from build123d import *

# Parameters (mm, degrees)
SKETCH_1_R               = 250
EXTRUDE_1_DEPTH          = 50
CHAMFER_1_SIZE           = 1
CUT_EXTRUDE_1_DEPTH      = 22
CUT_EXTRUDE_2_DEPTH      = 16
CUT_EXTRUDE_3_DEPTH      = 22
CUT_EXTRUDE_4_DEPTH      = 16
PATTERN_CIRCULAR_1_COUNT = 4
SKETCH_6_R               = 60
CUT_EXTRUDE_5_DEPTH      = 20
SKETCH_22_R              = 40
CUT_EXTRUDE_13_DEPTH     = 355.823899984


with BuildPart() as part:
    # Sketch 1 → Extrude 1 (new body)
    with BuildSketch(Plane(origin=(0, 0, 0), x_dir=(1, 0, 0), z_dir=(0, 1, 0))):
        with Locations(Location((0, 0, 0), (0, 0, 270))):
            Circle(SKETCH_1_R)
    extrude(amount=EXTRUDE_1_DEPTH)

    # Chamfer 1
    chamfer_1_edges = [part.edges().sort_by_distance(p)[0] for p in [
        (0, 0, -250),
        (0, 50, -250),
    ]]
    chamfer(chamfer_1_edges, length=CHAMFER_1_SIZE)

    # Sketch 2 → Cut-Extrude 1 (cut)
    with BuildSketch(Plane(origin=(0, 50, 0), x_dir=(1, 0, 0), z_dir=(0, 1, 0))):
        with BuildLine():
            Line((125, 11), (250, 11))
            Line((250, 11), (250, -11))
            Line((250, -11), (125, -11))
            ThreePointArc((125, -11), (114, 0), (125, 11))
        make_face()
    cut_extrude_1 = extrude(amount=-CUT_EXTRUDE_1_DEPTH, mode=Mode.SUBTRACT)

    # Sketch 3 → Cut-Extrude 2 (cut)
    with BuildSketch(Plane(origin=(0, 28, 0), x_dir=(1, 0, 0), z_dir=(0, 1, 0))):
        with BuildLine():
            Line((250, 19), (250, -19))
            Line((250, -19), (125, -19))
            ThreePointArc((125, -19), (106, 0), (125, 19))
            Line((125, 19), (250, 19))
        make_face()
    cut_extrude_2 = extrude(amount=-CUT_EXTRUDE_2_DEPTH, mode=Mode.SUBTRACT)

    # Sketch 4 → Cut-Extrude 3 (cut)
    with BuildSketch(Plane(origin=(0, 50, 0), x_dir=(1, 0, 0), z_dir=(0, 1, 0))):
        with BuildLine():
            Line((168.998520704, 184.55486989), (184.55486989, 168.998520704))
            Line((184.55486989, 168.998520704), (96.166522241, 80.610173055))
            ThreePointArc((96.166522241, 80.610173055), (80.610173055, 80.610173055), (80.610173055, 96.166522241))
            Line((80.610173055, 96.166522241), (168.998520704, 184.55486989))
        make_face()
    cut_extrude_3 = extrude(amount=-CUT_EXTRUDE_3_DEPTH, mode=Mode.SUBTRACT)

    # Sketch 5 → Cut-Extrude 4 (cut)
    with BuildSketch(Plane(origin=(0, 28, 0), x_dir=(1, 0, 0), z_dir=(0, 1, 0))):
        with BuildLine():
            Line((163.341666454, 190.211724139), (190.211724139, 163.341666454))
            Line((190.211724139, 163.341666454), (101.823376491, 74.953318806))
            ThreePointArc((101.823376491, 74.953318806), (74.953318806, 74.953318806), (74.953318806, 101.823376491))
            Line((74.953318806, 101.823376491), (163.341666454, 190.211724139))
        make_face()
    cut_extrude_4 = extrude(amount=-CUT_EXTRUDE_4_DEPTH, mode=Mode.SUBTRACT)

    # Pattern Circular 1: Cut-Extrude 1, Cut-Extrude 2, Cut-Extrude 3, Cut-Extrude 4 ×4 about axis
    pattern_circular_1_axis = Axis((0, 0, 0), (0, 1, 0))
    add([cut_extrude_1.rotate(pattern_circular_1_axis, i * 360 / PATTERN_CIRCULAR_1_COUNT) for i in range(1, PATTERN_CIRCULAR_1_COUNT)], mode=Mode.SUBTRACT)
    add([cut_extrude_2.rotate(pattern_circular_1_axis, i * 360 / PATTERN_CIRCULAR_1_COUNT) for i in range(1, PATTERN_CIRCULAR_1_COUNT)], mode=Mode.SUBTRACT)
    add([cut_extrude_3.rotate(pattern_circular_1_axis, i * 360 / PATTERN_CIRCULAR_1_COUNT) for i in range(1, PATTERN_CIRCULAR_1_COUNT)], mode=Mode.SUBTRACT)
    add([cut_extrude_4.rotate(pattern_circular_1_axis, i * 360 / PATTERN_CIRCULAR_1_COUNT) for i in range(1, PATTERN_CIRCULAR_1_COUNT)], mode=Mode.SUBTRACT)

    # Sketch 6 → Cut-Extrude 5 (cut)
    with BuildSketch(Plane(origin=(0, 50, 0), x_dir=(1, 0, 0), z_dir=(0, 1, 0))):
        with Locations(Location((0, 0, 0), (0, 0, 270))):
            Circle(SKETCH_6_R)
    extrude(amount=-CUT_EXTRUDE_5_DEPTH, mode=Mode.SUBTRACT)

    # Sketch 22 → Cut-Extrude 13 (cut, through all)
    with BuildSketch(Plane(origin=(0, 30, 0), x_dir=(1, 0, 0), z_dir=(0, 1, 0))):
        with Locations(Location((0, 0, 0), (0, 0, 270))):
            Circle(SKETCH_22_R)
    extrude(amount=-CUT_EXTRUDE_13_DEPTH, mode=Mode.SUBTRACT)


with BuildPart() as body_2:
    # Split Bodies 2: the piece on the far side of the plane
    add(part.part)
    split(bisect_by=Plane(origin=(0, 28, 0), x_dir=(0, 0, -1), z_dir=(0, -1, 0)), keep=Keep.BOTTOM)


with BuildPart() as part_1:
    add(part.part)

    # Split Bodies 2
    split(bisect_by=Plane(origin=(0, 28, 0), x_dir=(0, 0, -1), z_dir=(0, -1, 0)), keep=Keep.TOP)


solid = part_1.part
Read the model definition and answer for the solid it produces. Units are mm, in the model's axes. A direction names the side the tool comes from. Give positions to 0.01 mm unless a question says otherwise; leave off trailing zeros. Write each loop counter-clockwise with the first axis right and the second up, starting at its lowest first coordinate (ties: lowest second). Pieces come first, ordered by that corner, then holes. Notation, with made-up numbers: (-38.5, 17) - (20.5, 17) arc R11 ccw to (20.5, 36) - close; hole circle Ø10 at (43.25, -18.75). An arc over 180 degrees is marked (long way). Return JSON: item names as keys, results as strings.
Q1. A cutting plane is placed at A-A, the plane x = 0. Determine the outline of the cut face in (y, z), and give its area (3 significant figures).
Reply:
{"outline": "(0, -249) - (1, -250) - (12, -250) - (12, -106) - (28, -106) - (28, -40) - (0, -40) - close; (0, 40) - (28, 40) - (28, 106) - (12, 106) - (12, 250) - (1, 250) - (0, 249) - close", "area": "7,150 mm²"}
Q2. For a pull along Z with two mould halves and no side action, classify faces 6 (the face through (-19, 20, -186)), 7 (the face through (130, 12, 130)), 8 (the face through (0, 20, 106)) as released by +Z, released by -Z, zero draft, split by the parting line, or undercut.
Reply:
{"face 6": "zero draft", "face 7": "undercut", "face 8": "released by +Z"}
Q3. A cutting plane is placed at B-B, the plane z = 0. Determine the outline of the cut face in (x, y), and give its area (3 significant figures).
Reply:
{"outline": "(-250, 1) - (-249, 0) - (-40, 0) - (-40, 28) - (-106, 28) - (-106, 12) - (-250, 12) - close; (40, 0) - (249, 0) - (250, 1) - (250, 12) - (106, 12) - (106, 28) - (40, 28) - close", "area": "7,150 mm²"}
Q4. Given P1, Ø1.5, axis at x = -137, y = 10, coming from the +Z side; P2, Ø5, axis at y = 20, z = -210.5, coming from the -X side; P3, Ø2, axis at x = -161, y = 7, coming from the -Z side, each flat-ended and moving along its own axis, determine where each tip first touches the part or whether it passes through.
Reply:
{"P1": "z = 209.61", "P2": "x = -138.69", "P3": "z = -192.09"}
Q5. For faces 1 (the face through (130, 12, -130)), 2 (the face through (-39.05, 14.2, -8.67)), 3 (the face through (106, 20, 0)), 4 (the face through (-186, 20, 19)), 5 (the face through (0, 20, -106)), determine the directions among +Z, -Z, +X, -X, +Y, -Y from which every point of the face is accessible in a straight line to the end or side of a thin tool.
Reply:
{"face 1": "+Y", "face 2": "+Y, -Y", "face 3": "+X, +Y", "face 4": "-X, +Y", "face 5": "-Z, +Y"}
Q6. Consider line 1 along X through (y, z) = (20, 0); line 2 along Z through (x, y) = (-3, 9.5); line 3 along X through (y, z) = (10.5, 0). Determine where each line is inside the solid, lowest interval first. Write a range as [from, to].
Reply:
{"line 1": "[-106, -40], [40, 106]", "line 2": "[-249.98, -39.89], [39.89, 249.98]", "line 3": "[-250, -40], [40, 250]"}
